from build123d import *

# Parameters (mm, degrees)
ESBO_O1_W                = 65
ESBO_O1_H                = 20
RESSALTO_EXTRUS_O1_DEPTH = 2
ESBO_O2_W                = 61
ESBO_O2_H                = 14
RESSALTO_EXTRUS_O2_DEPTH = 2
ESBO_O3_W                = 59
ESBO_O3_H                = 12.003847287
CORTE_EXTRUS_O1_DEPTH    = 0.5
FILETE1_R                = 1


with BuildPart() as part:
    # Esboço1 → Ressalto-extrusão1 (new body)
    with BuildSketch(Plane(origin=(0, 0, 0), x_dir=(1, 0, 0), z_dir=(0, 1, 0))):
        with Locations((32.5, -10)):
            Rectangle(ESBO_O1_W, ESBO_O1_H)
    extrude(amount=RESSALTO_EXTRUS_O1_DEPTH)

    # Esboço2 → Ressalto-extrusão2 (add)
    with BuildSketch(Plane(origin=(0, 2, 0), x_dir=(1, 0, 0), z_dir=(0, 1, 0))):
        with Locations((32.5, -10)):
            Rectangle(ESBO_O2_W, ESBO_O2_H)
    extrude(amount=RESSALTO_EXTRUS_O2_DEPTH)

    # Esboço3 → Corte-extrusão1 (cut)
    with BuildSketch(Plane(origin=(0, 4, 0), x_dir=(1, 0, 0), z_dir=(0, 1, 0))):
        with Locations((32.5, -9.998076357)):
            Rectangle(ESBO_O3_W, ESBO_O3_H)
    extrude(amount=-CORTE_EXTRUS_O1_DEPTH, mode=Mode.SUBTRACT)

    # Filete1
    filete1_edges = [part.edges().sort_by_distance(p)[0] for p in [
        (65, 2, 10),
        (32.5, 2, 0),
        (0, 2, 10),
        (32.5, 2, 20),
    ]]
    fillet(filete1_edges, radius=FILETE1_R)


solid = part.part
Geometry check sheet. Reference: the model listing, model coordinates, mm. A direction names the side the tool comes from. Coordinates: 2 decimals unless noted, no trailing zeros. Loops run counter-clockwise (first coordinate to the right, second up) from the corner with the lowest first, then second, coordinate; pieces in that order, holes last. Notation, with made-up numbers: (10.25, 64) - (33.25, 64) arc R15 cw to (33.25, 89) - close; hole circle Ø3 at (27.25, 69). An arc over 180 degrees is marked (long way). Use one line per item in the form item = value. Start each with the question number.
Item 1: Gauge pin test, flat ends, axial feed: pin 1 (2 mm diameter, centred on y = 2.5, z = 12, fed in from -X); pin 2 (1.5 mm diameter, centred on x = 33, y = 3, fed in from -Z); pin 3 (1 mm diameter, centred on x = 38, y = 3, fed in from +Z). Record the tip position at first contact, or that the pin passes through.
Item 2: Section check B-B, the plane x = 59. Enter the section's corners in (y, z), and give its area (3 significant figures).
Item 3: Section check C-C, the plane y = 2.9. Enter the section's corners in (x, z), and give its area (3 significant figures).
Item 4: Tool access check on faces 1 (the face through (32, 0, 10)), 2 (the face through (32, 3, 3)), 3 (the face through (2, 3, 10)), 4 (the face through (32, 3, 17)). Record the directions out of +Z, -Z, +X, -X, +Y, -Y that give a thin tool (end or side, any length) a straight path to the whole face; none if there is none.
Item 5: Section check A-A, the plane z = 14. Enter the section's corners in (x, y).
Item 6: Mould release check, pull along X, two halves, no side actions. Record for faces 5 (the face through (27.8, 4, 16.2)), 6 (the face through (32, 3.5, 10)), 7 (the face through (63, 3, 10)): +X half, -X half, draft (parallel to the pull), parting line (faces both ways), or undercut.
Item 7: Thickness scan on probe 1 along Z at (x, y) = (25, 3.8); probe 2 along Y at (x, z) = (48, 9.25); probe 3 along Z at (x, y) = (16.5, 2.55). Record the ranges inside material, lowest first.
Computed:
q1.pin_1 = 0.13
q1.pin_2 = 3
q1.pin_3 = 17
q2.outline = (0, 0) - (1, 0) arc R1 ccw to (2, 1) - (2, 3) - (4, 3) - (4, 4) - (3.5, 4) - (3.5, 16) - (4, 16) - (4, 17) - (2, 17) - (2, 19) arc R1 ccw to (1, 20) - (0, 20) - close
q2.area = 61.6 mm2
q3.outline = (2, 3) - (63, 3) - (63, 17) - (2, 17) - close
q3.area = 854 mm2
q4.face_1 = +Z, -Z, +X, -X, -Y
q4.face_2 = -Z, +X, -X, +Y
q4.face_3 = +Z, -Z, -X, +Y
q4.face_4 = +Z, +X, -X, +Y
q5.outline = (0, 0) - (65, 0) - (65, 1) arc R1 ccw to (64, 2) - (63, 2) - (63, 4) - (62, 4) - (62, 3.5) - (3, 3.5) - (3, 4) - (2, 4) - (2, 2) - (1, 2) arc R1 ccw to (0, 1) - close
q6.face_5 = draft
q6.face_6 = undercut
q6.face_7 = +X half
q7.probe_1 = 3 to 4, 16 to 17
q7.probe_2 = 0 to 3.5
q7.probe_3 = 3 to 17
